The model under review builds one solid part; all positions refer to its coordinate system, in mm. Face numbers are marked on the shaded views. A direction names the side the tool comes from. Round coordinates to 2 decimals unless told otherwise and drop trailing zeros. Order: outer loops, then holes, each group sorted by start corner. A loop starts at its lowest first (then second) coordinate and runs counter-clockwise, first axis right, second up. Notation, with made-up numbers: M -1,89.25 L 36,89.25 A32 ccw 36,121.25 Z; hole C 0.5,78.5 d8. An arc over 180 degrees is marked long. Answer as a JSON object with one key per item and string values. Group by question number.
1) Consider section C-C, the plane y = -943.5. Write out the cut boundary in (x, z).
2) To check wall thickness, follow line 1 (Y direction, x = -58, z = 769.5); line 2 (X direction, y = -1487.5, z = 1441.5). State the ranges of each line that lie inside material, in increasing order.
3) Consider section B-B, the plane z = 157. Write out the cut boundary in (x, y).
4) Insertion check: pin 1 Ø1 at (x, z) = (-13, 1545.5) entering from -Y; pin 2 Ø1.5 at (y, z) = (-267.5, 516) entering from +X; pin 3 Ø2 at (y, z) = (-494.5, 1220.5) entering from -X. Each pin has a flat end and moves straight along its axis. Give the tip position at first contact, or say it passes through.
5) For the marked faces 1, 2 and 3, list the 3-axis set-ups (+Z, -Z, +X, -X, +Y, -Y) from which the entire face can be reached by the end or side of a thin tool; tool diameter is ignored.
6) Consider section A-A, the plane x = -133.5. Write out the cut boundary in (y, z).
7) Consider section D-D, the plane x = -5. Write out the cut boundary in (y, z).
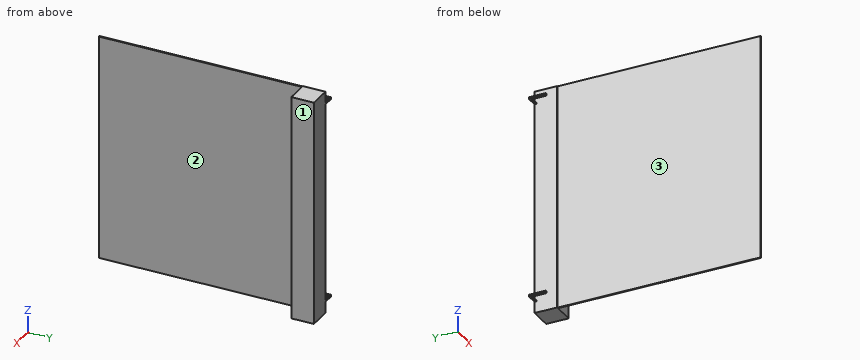
Autodesk Inventor part; units mm, degrees
ref_plane "YZ Plane" through (0, 0, 0) normal (1, 0, 0) x (0, 1, 0)
ref_plane "XZ Plane" through (0, 0, 0) normal (0, 1, 0) x (-1, 0, 0)
ref_plane "XY Plane" through (0, 0, 0) normal (0, 0, 1) x (1, 0, 0)
sketch "Esquisse1" plane through (0, 0, 0) normal (0, 0, 1) x (1, 0, 0)
  line L0 (-100, 100) -> (100, 100)
  line L1 (100, 100) -> (100, -100)
  line L2 (100, -100) -> (-100, -100)
  line L3 (-100, -100) -> (-100, 100)
  line L4 (-95.2971, -100) -> (-85.2971, -100)
  line L5 (-85.2971, -100) -> (-85.2971, -1900)
  line L6 (-85.2971, -1900) -> (-95.2971, -1900)
  line L7 (-95.2971, -1900) -> (-95.2971, -100)
  point P0 (0, 0)
  dimension "d0" = 200
  dimension "d1" = 200
  dimension "d2" = 100
  dimension "d3" = 100
  dimension "d4" = 1800
  dimension "d5" = 10
extrude "Extrusion1" add sketch "Esquisse1" along normal blind 2000
sketch "Esquisse2" plane through (-100, 100, 0) normal (0, 1, 0) x (1, 0, 0)
  line L0 (14.7029, 0) -> (14.7029, -2000)
  line L1 (14.7029, -1926.0048) -> (14.7029, -1942.8259)
  line L2 (4.7029, 0) -> (4.7029, -2000)
  line L3 (4.7029, -126.1575) -> (4.7029, -105.1313)
  line L4 (0, 0) -> (0, -2000)
  line L5 (0, -1900) -> (-100, -1900)
  line L6 (-100, -1900) -> (-100, -1885)
  line L7 (-100, -1885) -> (0, -1885)
  line L8 (0, -1885) -> (0, -1900)
  line L9 (0, -115) -> (-100, -115)
  line L10 (-100, -115) -> (-100, -100)
  line L11 (-100, -100) -> (0, -100)
  line L12 (0, -100) -> (0, -115)
  point P0 (100, 0)
  dimension "d8" = 100
  dimension "d9" = 15
  dimension "d10" = 100
  dimension "d11" = 100
  dimension "d12" = 15
  dimension "d13" = 100
extrude "Extrusion2" add sketch "Esquisse2" against normal blind 150
sketch "Esquisse3" plane through (-200, 100, 1900) normal (0, 0, 1) x (1, 0, 0)
  line L0 (0, -150) -> (100, -150)
  line L1 (100, 0) -> (100, -200)
  line L2 (15, -150) -> (100, -150)
  line L3 (100, -150) -> (100, -15)
  line L4 (100, -15) -> (15, -15)
  line L5 (15, -15) -> (15, -150)
  line L6 (0, 0) -> (100, 0)
  point P0 (200, -100)
  dimension "d16" = 15
  dimension "d17" = 15
extrude "Extrusion3" cut sketch "Esquisse3" against normal through all
properties part number "Ecran_Videoprojecteur"
Results list:
{
 "1": {"outline": "M -95.3,0 L -85.3,0 L -85.3,2000 L -95.3,2000 Z"},
 "2": {"line 1": "-100 to 100", "line 2": "-95.3 to -85.3"},
 "3": {"outline": "M -100,-100 L -95.3,-100 L -95.3,-1900 L -85.3,-1900 L -85.3,-100 L 100,-100 L 100,100 L -100,100 Z"},
 "4": {"pin 1": "y = -100", "pin 2": "x = -85.3", "pin 3": "x = -95.3"},
 "5": {"face 1": "+Z, -Z, +X, +Y, -Y", "face 2": "+Z, -Z, +X, -Y", "face 3": "+Z, -Z, -X, -Y"},
 "6": {"outline": "M 85,100 L 100,100 L 100,115 L 85,115 Z; M 85,1885 L 100,1885 L 100,1900 L 85,1900 Z"},
 "7": {"outline": "M -100,0 L 100,0 L 100,2000 L -100,2000 Z"}
}
